from build123d import *

# Parameters (mm, degrees)
F0_W     = 76.2
F0_H     = 19.05
F1_DEPTH = 2.54
F2_W     = 3.81
F2_H     = 19.05
F3_DEPTH = 10.16
F4_R     = 4.445
F5_DEPTH = 25.4
F7_DEPTH = 19.05


with BuildPart() as f1:
    # F0 (on Top) → F1 (new body)
    with BuildSketch(Plane.XY):
        with Locations((38.1, 9.525)):
            Rectangle(F0_W, F0_H)
    extrude(amount=F1_DEPTH)

    # F2 (on face) → F3 (join)
    with BuildSketch(Plane.XY.offset(2.54)):
        with Locations((1.905, 9.525)):
            Rectangle(F2_W, F2_H)
        with Locations((74.295, 9.525)):
            Rectangle(F2_W, F2_H)
    extrude(amount=F3_DEPTH)

    # F4 (on face) → F5 (cut)
    with BuildSketch(Plane.XY.offset(2.54)):
        with Locations((38.1, 9.525)):
            Circle(F4_R)
    extrude(amount=-F5_DEPTH, mode=Mode.SUBTRACT)

    # F6 (on face) → F7 (join, through all)
    with BuildSketch(Plane.XZ):
        Polygon((0, 8.89), (0, 12.7), (-1.27, 12.7), align=None)
        Polygon((76.2, 12.7), (76.2, 8.89), (77.47, 12.7), align=None)
    extrude(amount=-F7_DEPTH)


solid = f1.part
Can you work these out from the model? Positions are in its coordinate system, mm. A direction names the side the tool comes from. Give positions to 0.01 mm unless a question says otherwise; leave off trailing zeros. Write each loop counter-clockwise with the first axis right and the second up, starting at its lowest first coordinate (ties: lowest second). Pieces come first, ordered by that corner, then holes. Notation, with made-up numbers: (21, 89.25) -> (45, 89.25) arc R17 ccw to (45, 114.25) -> close; hole circle Ø3 at (27.25, 86). An arc over 180 degrees is marked (long way). Answer as a JSON object with one key per item and string values. Group by question number.
Item 1: We'd pull the mould along X, two halves only. Please class faces 4 (the face through (76.826, 9.392, 10.768)), 5 (the face through (38, 0, 2)), 6 (the face through (42.34, 10.86, 1.29)): +X half, -X half, draft (parallel to the pull), parting line (faces both ways), or undercut.
Item 2: Suppose I cut it at D-D (x = 51). Please give me the cut outline in (y, z), plus the area to 3 significant figures.
Item 3: Please list where these lines run through material, in increasing order: line 1 (X direction, y = 16.25, z = 4.25); line 2 (Y direction, x = 38.1, z = 1.6); line 3 (Z direction, x = 55, y = 11.75). Write a range as [from, to].
Item 4: Suppose I cut it at B-B (x = 38.1). Please give me the cut outline in (y, z), plus the area to 3 significant figures.
Item 5: Suppose I cut it at A-A (z = 6). Please give me the cut outline in (x, y).
Item 6: I'm going to push flat-ended pins straight in: P1, Ø5, axis at y = 7.5, z = 7.5, coming from the +X side; P2, Ø5, axis at x = 37, z = 6.5, coming from the -Y side; P3, Ø8, axis at x = 10, y = 11, coming from the +Z side; P4, Ø2.5, axis at y = 6, z = 5, coming from the -X side. Where does each tip first touch, or does it pass through?
Item 7: Suppose I cut it at C-C (y = 2.75). Please give me the cut outline in (x, z).
Item 8: For faces 1 (the face through (76.2, 9, 4)), 2 (the face through (38, 16, 2.54)), 3 (the face through (0, 9, 4)), which set-ups out of +Z, -Z, +X, -X, +Y, -Y let a thin tool reach every point of the face, with its end or its side?
Findings:
{
 "1": {"face 4": "+X half", "face 5": "draft", "face 6": "undercut"},
 "2": {"outline": "(0, 0) -> (19.05, 0) -> (19.05, 2.54) -> (0, 2.54) -> close", "area": "48.4 mm²"},
 "3": {"line 1": "x = [0, 3.81], [72.39, 76.2]", "line 2": "y = [0, 5.08], [13.97, 19.05]", "line 3": "z = [0, 2.54]"},
 "4": {"outline": "(0, 0) -> (5.08, 0) -> (5.08, 2.54) -> (0, 2.54) -> close; (13.97, 0) -> (19.05, 0) -> (19.05, 2.54) -> (13.97, 2.54) -> close", "area": "25.8 mm²"},
 "5": {"outline": "(0, 0) -> (3.81, 0) -> (3.81, 19.05) -> (0, 19.05) -> close; (72.39, 0) -> (76.2, 0) -> (76.2, 19.05) -> (72.39, 19.05) -> close"},
 "6": {"P1": "stops at x = 76.57", "P2": "passes through", "P3": "stops at z = 2.54", "P4": "stops at x = 0"},
 "7": {"outline": "(-1.27, 12.7) -> (0, 8.89) -> (0, 0) -> (76.2, 0) -> (76.2, 8.89) -> (77.47, 12.7) -> (72.39, 12.7) -> (72.39, 2.54) -> (3.81, 2.54) -> (3.81, 12.7) -> close"},
 "8": {"face 1": "-Z, +X, +Y, -Y", "face 2": "+Z, +Y, -Y", "face 3": "-Z, -X, +Y, -Y"}
}
